from build123d import *

# Parameters (mm, degrees)
SKETCH_1_W          = 36
SKETCH_1_H          = 36
EXTRUDE_1_DEPTH     = 1
FILLET_1_R          = 3
SKETCH_2_R          = 1.5
CUT_EXTRUDE_1_DEPTH = 1


with BuildPart() as part:
    # 草图1 → 凸台-拉伸1 (new body)
    with BuildSketch(Plane.XY):
        Rectangle(SKETCH_1_W, SKETCH_1_H)
    extrude(amount=EXTRUDE_1_DEPTH)

    # 圆角1
    fillet_1_edges = [part.edges().sort_by_distance(p)[0] for p in [
        (-18, 18, 0.5),
        (18, 18, 0.5),
        (18, -18, 0.5),
        (-18, -18, 0.5),
    ]]
    fillet(fillet_1_edges, radius=FILLET_1_R)

    # 草图2 → 切除-拉伸1 (cut)
    with BuildSketch(Plane.XY.offset(1)):
        with Locations((-15.25, 15.25)):
            Circle(SKETCH_2_R)
        with Locations((15.25, 15.25)):
            Circle(SKETCH_2_R)
        with Locations((15.25, -15.25)):
            Circle(SKETCH_2_R)
        with Locations((-15.25, -15.25)):
            Circle(SKETCH_2_R)
    extrude(amount=-CUT_EXTRUDE_1_DEPTH, mode=Mode.SUBTRACT)


solid = part.part
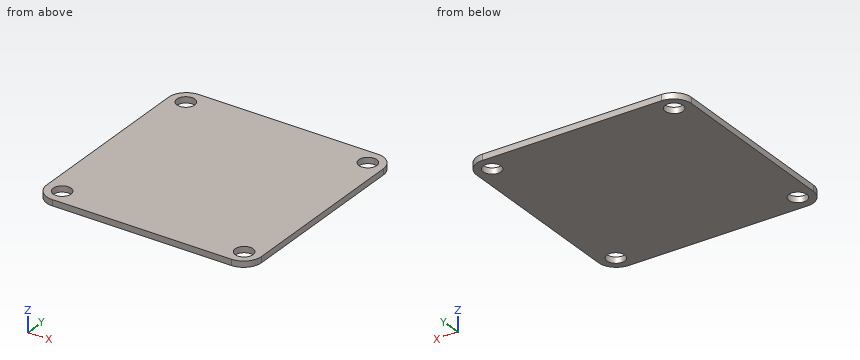
Could you check a few things on this model? Use its own coordinates, in mm. Give positions to 0.01 mm unless a question says otherwise; leave off trailing zeros. Order: outer loops, then holes, each group sorted by start corner. A loop starts at its lowest first (then second) coordinate and runs counter-clockwise, first axis right, second up. Notation, with made-up numbers: (36.5, 23) -> (59.5, 23) arc R19 ccw to (59.5, 44) -> close; hole circle Ø3 at (30, 14.25). An arc over 180 degrees is marked (long way). Return JSON: item names as keys, results as strings.
1. Imagine slicing it at C-C on x = -16. List the corners of the cut face in (y, z) for me, then the cut area to 3 significant figures.
Answer list:
{"outline": "(-17.83, 0) -> (-16.55, 0) -> (-16.55, 1) -> (-17.83, 1) -> close; (-13.95, 0) -> (13.95, 0) -> (13.95, 1) -> (-13.95, 1) -> close; (16.55, 0) -> (17.83, 0) -> (17.83, 1) -> (16.55, 1) -> close", "area": "30.5 mm2"}
2. For pin 1 Ø2.5 at (x, y) = (15.25, -15.25) entering from +Z, with a flat end and sliding along its axis, tell me the tip position at first contact or that it passes through.
Answer list:
{"pin 1": "passes through"}
3. I need wall thicknesses on line 1 (Y direction, x = -15.25, z = 0.75); line 2 (X direction, y = 14, z = 0.8). Which ranges of each line are inside material? Lowest first, please. Write a range as from..to.
Answer list:
{"line 1": "y = -17.99..-16.75, -13.75..13.75, 16.75..17.99", "line 2": "x = -18..-16.08, -14.42..14.42, 16.08..18"}
4. Imagine slicing it at A-A on z = 0.55. List the corners of the cut face in (x, y) for me, then the cut area to 3 significant figures.
Answer list:
{"outline": "(-18, -15) arc R3 ccw to (-15, -18) -> (15, -18) arc R3 ccw to (18, -15) -> (18, 15) arc R3 ccw to (15, 18) -> (-15, 18) arc R3 ccw to (-18, 15) -> close; hole circle Ø3 at (-15.25, -15.25); hole circle Ø3 at (-15.25, 15.25); hole circle Ø3 at (15.25, -15.25); hole circle Ø3 at (15.25, 15.25)", "area": "1,260 mm2"}
5. Imagine slicing it at B-B on x = 14.5. List the corners of the cut face in (y, z) for me, then the cut area to 3 significant figures.
Answer list:
{"outline": "(-18, 0) -> (-16.55, 0) -> (-16.55, 1) -> (-18, 1) -> close; (-13.95, 0) -> (13.95, 0) -> (13.95, 1) -> (-13.95, 1) -> close; (16.55, 0) -> (18, 0) -> (18, 1) -> (16.55, 1) -> close", "area": "30.8 mm2"}
